Read the model definition and answer for the solid it produces. Units are mm, in the model's axes. A direction names the side the tool comes from. Give positions to 0.01 mm unless a question says otherwise; leave off trailing zeros. Write each loop counter-clockwise with the first axis right and the second up, starting at its lowest first coordinate (ties: lowest second). Pieces come first, ordered by that corner, then holes. Notation, with made-up numbers: (-26.75, 8) - (23.25, 8) arc R23 ccw to (23.25, 31) - close; hole circle Ø10 at (11.25, 38.25). An arc over 180 degrees is marked (long way). Answer as a JSON object with one key per item and string values. Group by question number.
```python
from build123d import *

# Parameters (mm, degrees)
SKETCH_R          = 42.0538238692
SKETCH_R_2        = 23
SKETCH_R_3        = 2.6
PAD_DEPTH         = 4
SKETCH001_R       = 25
SKETCH001_R_2     = 23
PAD001_DEPTH      = 50
POCKET_DEPTH      = 25
POCKET_DEPTH_BACK = 25
SKETCH003_R       = 31
PAD002_DEPTH      = 3
SKETCH004_R       = 42.0538238692
SKETCH004_R_2     = 25
POCKET001_DEPTH   = 55
SKETCH005_R       = 2.7
POCKET002_DEPTH   = 5
SKETCH006_W       = 30
SKETCH006_H       = 20
POCKET003_DEPTH   = 25.5
PAD003_DEPTH      = 3
SKETCH008_W       = 50
SKETCH008_H       = 10
POCKET004_DEPTH   = 7
FILLET_R          = 2
CHAMFER_SIZE      = 1
CHAMFER001_SIZE   = 2.5


with BuildPart() as part:
    # Sketch → Pad (new body)
    with BuildSketch(Plane.XY):
        Circle(SKETCH_R)
        Circle(SKETCH_R_2, mode=Mode.SUBTRACT)
        with Locations((-23, 23)):
            Circle(SKETCH_R_3, mode=Mode.SUBTRACT)
        with Locations((23, 23)):
            Circle(SKETCH_R_3, mode=Mode.SUBTRACT)
        with Locations((23, -23)):
            Circle(SKETCH_R_3, mode=Mode.SUBTRACT)
        with Locations((-23, -23)):
            Circle(SKETCH_R_3, mode=Mode.SUBTRACT)
    extrude(amount=PAD_DEPTH)

    # Sketch001 (on Face8 of Pad) → Pad001 (join)
    with BuildSketch(Plane.XY.offset(4)):
        Circle(SKETCH001_R)
        Circle(SKETCH001_R_2, mode=Mode.SUBTRACT)
    extrude(amount=PAD001_DEPTH)

    # Sketch002 → Pocket (cut, two sides)
    with BuildSketch(Plane.YZ) as pocket_sk:
        Polygon((-25, 54), (25, 25.1324865414), (25, 54), align=None)
    extrude(amount=-POCKET_DEPTH, mode=Mode.SUBTRACT)
    extrude(pocket_sk.sketch, amount=POCKET_DEPTH_BACK, mode=Mode.SUBTRACT)

    # Sketch003 (on Face11 of Pocket) → Pad002 (join)
    with BuildSketch(Plane(origin=(0, 17.1326859021, 29.6746824535), x_dir=(1, 0, 0), z_dir=(0, 0.5, 0.8660254038))):
        with Locations((0, -19.7831216349)):
            Circle(SKETCH003_R)
    extrude(amount=PAD002_DEPTH)

    # Sketch004 (on Face5 of Pad002) → Pocket001 (cut)
    with BuildSketch(Plane.XY.offset(4)):
        Circle(SKETCH004_R)
        Circle(SKETCH004_R_2, mode=Mode.SUBTRACT)
    extrude(amount=POCKET001_DEPTH, mode=Mode.SUBTRACT)

    # Sketch005 (on Face13 of Pocket001) → Pocket002 (cut)
    with BuildSketch(Plane(origin=(0, 17.1326859021, 29.6746824535), x_dir=(1, 0, 0), z_dir=(0, -0.5, -0.8660254038))):
        with Locations((-8, 12)):
            Circle(SKETCH005_R)
        with Locations((8, 12)):
            Circle(SKETCH005_R)
    extrude(amount=-POCKET002_DEPTH, mode=Mode.SUBTRACT)

    # Sketch006 → Pocket003 (cut, symmetric)
    with BuildSketch(Plane.YZ):
        with Locations((-15, 53.0303448858)):
            Rectangle(SKETCH006_W, SKETCH006_H)
    extrude(amount=POCKET003_DEPTH, both=True, mode=Mode.SUBTRACT)

    # Sketch007 (on Face4 of Pocket003) → Pad003 (join)
    with BuildSketch(Plane.XY.offset(43.0303448858)):
        with BuildLine():
            ThreePointArc((-25, 0), (0, -25), (25, 0))
            Line((-25, 0), (25, 0))
        make_face()
    extrude(amount=PAD003_DEPTH)

    # Sketch008 (on Face13 of Pad003) → Pocket004 (cut)
    with BuildSketch(Plane(origin=(0, 18.6326859021, 32.2727586649), x_dir=(1, 0, 0), z_dir=(0, 0.5, 0.8660254038))):
        with Locations((0, -26.5151724424)):
            Rectangle(SKETCH008_W, SKETCH008_H)
    extrude(amount=POCKET004_DEPTH, mode=Mode.SUBTRACT)

    # Fillet
    fillet_edges = [part.edges().sort_by_distance(p)[0] for p in [
        (-23, 0, 0),
        (-42.053824, 0, 0),
        (0, -25, 46.030345),
    ]]
    fillet(fillet_edges, radius=FILLET_R)

    # Chamfer
    chamfer_edges = [part.edges().sort_by_distance(p)[0] for p in [
        (5.3, 6.740381, 35.674682),
        (-10.7, 6.740381, 35.674682),
    ]]
    chamfer(chamfer_edges, length=CHAMFER_SIZE)

    # Chamfer001
    chamfer001_edges = [part.edges().sort_by_distance(p)[0] for p in [
        (20.4, -23, 0),
        (20.4, 23, 0),
        (-25.6, 23, 0),
        (-25.6, -23, 0),
    ]]
    chamfer(chamfer001_edges, length=CHAMFER001_SIZE)


solid = part.part
```
1) For a pull along X with two mould halves and no side action, classify faces 1 (the conical face through (20.968, 24.863, 2.344)), 2 (the flat face through (0, -12, 46.03)), 3 (the cylindrical face through (-5.475, 41.696, 2.986)) as released by +X, released by -X, zero draft, split by the parting line, or undercut.
2) Which of the six approach directions +Z, -Z, +X, -X, +Y, -Y give full straight-line access (tool end or side, diameter ignored) to faces 4 (the cylindrical face through (-4.986, -22.453, 17.669)), 5 (the cylindrical face through (-5.42, -24.406, 23.735)), 6 (the flat face through (-18.4, -17.2, 0))?
3) Find section C-C, the plane y = 0. Write down the section's boundary in (x, z).
4) Find section A-A, the plane x = 0. Write down the section's boundary in (y, z), and give its area (3 significant figures).
5) Flat-ended cylindrical pins translate along their axes: pin 1 Ø3 at (y, z) = (4, 6) entering from +X; pin 2 Ø8.5 at (x, y) = (-23, 23) entering from +Z; pin 3 Ø8 at (x, z) = (-17, 25) entering from +Y; pin 4 Ø4 at (y, z) = (-28, 35.5) entering from +X. Find the tip coordinate at first contact, or state that the pin passes through.
6) Find section B-B, the plane z = 20.5. Write down the section's boundary in (x, y).
7) Find the intervals of material crossed by line 1 (X direction, y = 13, z = 18); line 2 (Y direction, x = 0, z = 18); line 3 (X direction, y = -2.5, z = 27), in increasing order. Write a range as [from, to].
Values follow:
{
 "1": {"face 1": "undercut", "face 2": "zero draft", "face 3": "split by the parting line"},
 "2": {"face 4": "-Z", "face 5": "+Z", "face 6": "-Z, +X, -X, +Y, -Y"},
 "3": {"outline": "(-42.05, 2) arc R2 ccw to (-40.05, 0) - (-25, 0) arc R2 ccw to (-23, 2) - (-23, 39.57) - (23, 39.57) - (23, 2) arc R2 ccw to (25, 0) - (40.05, 0) arc R2 ccw to (42.05, 2) - (42.05, 4) - (25, 4) - (25, 43.03) - (-25, 43.03) - (-25, 4) - (-42.05, 4) - close"},
 "4": {"outline": "(-42.05, 2) arc R2 ccw to (-40.05, 0) - (-25, 0) arc R2 ccw to (-23, 2) - (-23, 43.03) - (-6, 43.03) - (23, 26.29) - (23, 2) arc R2 ccw to (25, 0) - (40.05, 0) arc R2 ccw to (42.05, 2) - (42.05, 4) - (25, 4) - (25, 28.6) - (-5.2, 46.03) - (-23, 46.03) arc R2 ccw to (-25, 44.03) - (-25, 4) - (-42.05, 4) - close", "area": "434 mm2"},
 "5": {"pin 1": "stops at x = 24.87", "pin 2": "stops at z = 4", "pin 3": "stops at y = 21.35", "pin 4": "passes through"},
 "6": {"outline": "circle Ø50 at (0, 0); hole circle Ø46 at (0, 0)"},
 "7": {"line 1": "x = [-21.35, -18.97], [18.97, 21.35]", "line 2": "y = [-25, -23], [23, 25]", "line 3": "x = [-24.87, -22.86], [22.86, 24.87]"}
}
